from build123d import *

# Parameters (mm, degrees)
BOSS_EXTRUDE1_DEPTH = 12
BOSS_EXTRUDE2_DEPTH = 9
BOSS_EXTRUDE3_DEPTH = 12
SKETCH1_5_R         = 52.5
SKETCH1_5_R_2       = 40.5
BOSS_EXTRUDE4_DEPTH = 63
SKETCH1_6_R         = 23.665
SKETCH1_6_R_2       = 11.665
BOSS_EXTRUDE5_DEPTH = 25


with BuildPart() as part:
    # Sketch1 → Boss-Extrude1 (new body)
    with BuildSketch(Plane(origin=(0, 0, 0), x_dir=(1, 0, 0), z_dir=(0, 1, 0))):
        with BuildLine():
            Line((95.298631714, 22.343087709), (17.301, 49.56738241))
            ThreePointArc((17.301, 49.56738241), (42.805096075, 30.396936523), (52.5, 0))
            ThreePointArc((52.5, 0), (42.805096075, -30.396936523), (17.301, -49.56738241))
            Line((17.301, -49.56738241), (95.298631714, -22.343087709))
            ThreePointArc((95.298631714, -22.343087709), (63.835, 0), (95.298631714, 22.343087709))
        make_face()
        with BuildLine():
            Line((71.809327621, -27.364302024), (49.82603874, -35.037349549))
            ThreePointArc((49.82603874, -35.037349549), (46.470783868, -34.048587089), (46.332927596, -30.553392944))
            ThreePointArc((46.332927596, -30.553392944), (55.5, 0), (46.332927596, 30.553392944))
            ThreePointArc((46.332927596, 30.553392944), (46.470783868, 34.048587089), (49.82603874, 35.037349549))
            Line((49.82603874, 35.037349549), (71.809327621, 27.364302024))
            ThreePointArc((71.809327621, 27.364302024), (73.795133067, 24.922702734), (72.507464694, 22.050988869))
            ThreePointArc((72.507464694, 22.050988869), (60.835, 0), (72.507464694, -22.050988869))
            ThreePointArc((72.507464694, -22.050988869), (73.795133067, -24.922702734), (71.809327621, -27.364302024))
        make_face(mode=Mode.SUBTRACT)
    extrude(amount=BOSS_EXTRUDE1_DEPTH)

    # Sketch1_3 → Boss-Extrude2 (add)
    with BuildSketch(Plane(origin=(0, 0, 0), x_dir=(1, 0, 0), z_dir=(0, 1, 0))):
        with BuildLine():
            ThreePointArc((49.82603874, -35.037349549), (46.470783868, -34.048587089), (46.332927596, -30.553392944))
            ThreePointArc((46.332927596, -30.553392944), (55.5, 0), (46.332927596, 30.553392944))
            ThreePointArc((46.332927596, 30.553392944), (46.470783868, 34.048587089), (49.82603874, 35.037349549))
            Line((49.82603874, 35.037349549), (71.809327621, 27.364302024))
            ThreePointArc((71.809327621, 27.364302024), (73.795133067, 24.922702734), (72.507464694, 22.050988869))
            ThreePointArc((72.507464694, 22.050988869), (60.835, 0), (72.507464694, -22.050988869))
            ThreePointArc((72.507464694, -22.050988869), (73.795133067, -24.922702734), (71.809327621, -27.364302024))
            Line((71.809327621, -27.364302024), (49.82603874, -35.037349549))
        make_face()
        with BuildLine():
            ThreePointArc((-46.332927596, 30.553392944), (-55.5, 0), (-46.332927596, -30.553392944))
            ThreePointArc((-46.332927596, -30.553392944), (-46.470783868, -34.048587089), (-49.82603874, -35.037349549))
            Line((-49.82603874, -35.037349549), (-71.809327621, -27.364302024))
            ThreePointArc((-71.809327621, -27.364302024), (-73.795133067, -24.922702734), (-72.507464694, -22.050988869))
            ThreePointArc((-72.507464694, -22.050988869), (-60.835, 0), (-72.507464694, 22.050988869))
            ThreePointArc((-72.507464694, 22.050988869), (-73.795133067, 24.922702734), (-71.809327621, 27.364302024))
            Line((-71.809327621, 27.364302024), (-49.82603874, 35.037349549))
            ThreePointArc((-49.82603874, 35.037349549), (-46.470783868, 34.048587089), (-46.332927596, 30.553392944))
        make_face()
    extrude(amount=BOSS_EXTRUDE2_DEPTH)

    # Sketch1_4 → Boss-Extrude3 (add)
    with BuildSketch(Plane(origin=(0, 0, 0), x_dir=(1, 0, 0), z_dir=(0, 1, 0))):
        with BuildLine():
            Line((-37.609789084, 42.478802323), (-95.298631714, 22.343087709))
            ThreePointArc((-95.298631714, 22.343087709), (-73.798218994, 19.29490664), (-63.835, 0))
            ThreePointArc((-63.835, 0), (-73.798218994, -19.29490664), (-95.298631714, -22.343087709))
            Line((-95.298631714, -22.343087709), (-17.301, -49.56738241))
            ThreePointArc((-17.301, -49.56738241), (-52.498391324, -0.410984604), (-18.074910259, 49.290441458))
            Line((-18.074910259, 49.290441458), (-37.609789084, 42.478802323))
        make_face()
        with BuildLine():
            ThreePointArc((-72.507464694, 22.050988869), (-73.795133067, 24.922702734), (-71.809327621, 27.364302024))
            Line((-71.809327621, 27.364302024), (-49.82603874, 35.037349549))
            ThreePointArc((-49.82603874, 35.037349549), (-46.470783868, 34.048587089), (-46.332927596, 30.553392944))
            ThreePointArc((-46.332927596, 30.553392944), (-55.5, 0), (-46.332927596, -30.553392944))
            ThreePointArc((-46.332927596, -30.553392944), (-46.470783868, -34.048587089), (-49.82603874, -35.037349549))
            Line((-49.82603874, -35.037349549), (-71.809327621, -27.364302024))
            ThreePointArc((-71.809327621, -27.364302024), (-73.795133067, -24.922702734), (-72.507464694, -22.050988869))
            ThreePointArc((-72.507464694, -22.050988869), (-60.835, 0), (-72.507464694, 22.050988869))
        make_face(mode=Mode.SUBTRACT)
    extrude(amount=BOSS_EXTRUDE3_DEPTH)

    # Sketch1_5 → Boss-Extrude4 (add)
    with BuildSketch(Plane(origin=(0, 0, 0), x_dir=(1, 0, 0), z_dir=(0, 1, 0))):
        Circle(SKETCH1_5_R)
        Circle(SKETCH1_5_R_2, mode=Mode.SUBTRACT)
    extrude(amount=BOSS_EXTRUDE4_DEPTH)

    # Sketch1_6 → Boss-Extrude5 (add)
    with BuildSketch(Plane(origin=(0, 0, 0), x_dir=(1, 0, 0), z_dir=(0, 1, 0))):
        with Locations((-87.5, 0)):
            Circle(SKETCH1_6_R)
        with Locations((-87.5, 0)):
            Circle(SKETCH1_6_R_2, mode=Mode.SUBTRACT)
        with Locations((87.5, 0)):
            Circle(SKETCH1_6_R)
        with Locations((87.5, 0)):
            Circle(SKETCH1_6_R_2, mode=Mode.SUBTRACT)
    extrude(amount=BOSS_EXTRUDE5_DEPTH)


solid = part.part
For this review, take the finished solid that the model builds, in its own axes (mm). A direction names the side the tool comes from. Give positions to 0.01 mm unless a question says otherwise; leave off trailing zeros. Loops run counter-clockwise (first coordinate to the right, second up) from the corner with the lowest first, then second, coordinate; pieces in that order, holes last. Notation, with made-up numbers: (65, 15) - (122, 15) arc R13 cw to (122, 32) - close; hole circle Ø5 at (35, 2). An arc over 180 degrees is marked (long way). Write each question's results on one line, items separated by ' | '.
(1) For line 1 along X through (y, z) = (18, 0) (3 decimals); line 2 along Z through (x, y) = (1, 17); line 3 along Z through (x, y) = (87.5, 15.25) (3 decimals), list the stretches that pass through material, from the lowest coordinate up.
Conclusion:
line 1: -111.165 to -99.165, -75.835 to -63.835, -52.5 to -40.5, 40.5 to 52.5, 63.835 to 75.835, 99.165 to 111.165 | line 2: -52.49 to -40.49, 40.49 to 52.49 | line 3: -23.665 to -11.665, 11.665 to 23.665
(2) For pin 1 Ø8 at (x, y) = (21, 33) entering from -Z; pin 2 Ø14 at (x, z) = (-58, 12) entering from +Y; pin 3 Ø23.5 at (x, z) = (-77.5, -6) entering from +Y; pin 4 Ø1.5 at (x, y) = (64.5, 7) entering from -Z, all flat-tipped, find the tip position at first contact; note any pin that passes through.
Conclusion:
pin 1: z = -49.67 | pin 2: y = 63 | pin 3: y = 25 | pin 4: z = -33.35
(3) Take a section at B-B (x = 0). Give the boundary of the cut face in (y, z).
Conclusion:
outline: (0, -52.5) - (63, -52.5) - (63, -40.5) - (0, -40.5) - close; (0, 40.5) - (63, 40.5) - (63, 52.5) - (0, 52.5) - close
(4) Take a section at A-A (z = 0). State how many separate pieces and enclosed holes the cut face has, then the cut area to 3 significant figures.
Conclusion:
separate pieces: 4 | enclosed holes: 0 | area: 2,950 mm^2
(5) For faces 5 (the flat face through (-60.664, 10.479, 31.255)), 6 (the flat face through (27, 63, 31)), list the 3-axis set-ups (+Z, -Z, +X, -X, +Y, -Y) from which the entire face can be reached by the end or side of a thin tool; tool diameter is ignored.
Conclusion:
face 5: +Y | face 6: +Z, -Z, +X, -X, +Y
(6) Draft analysis for pull direction X (two halves, no side actions). For faces 1 (the cylindrical face through (46.503, 10.479, 34.09)), 2 (the flat face through (55.754, 5.916, 36.146)), 3 (the cylindrical face through (-82.12, 12.32, 10.35)), 4 (the flat face through (-98.3, 25, 4.9)), state which applies: +X half, -X half, draft (parallel to the pull), parting line (faces both ways), or undercut.
Conclusion:
face 1: undercut | face 2: +X half | face 3: undercut | face 4: draft
(7) Take a section at C-C (y = 40.5). Give the boundary of the cut face in (x, z), then the cut area to 3 significant figures.
Conclusion:
outline: circle Ø105 at (0, 0); hole circle Ø81 at (0, 0) | area: 3,510 mm^2
(8) Take a section at D-D (x = -81). Give the boundary of the cut face in (y, z).
Conclusion:
outline: (0, -27.33) - (12, -27.33) - (12, -22.75) - (25, -22.75) - (25, -9.69) - (0, -9.69) - close; (0, 9.69) - (25, 9.69) - (25, 22.75) - (12, 22.75) - (12, 27.33) - (0, 27.33) - close
